CAD build for the part. Positions are in the model's coordinates, mm. Coordinates: 2 decimals unless noted, no trailing zeros. Loops run counter-clockwise (first coordinate to the right, second up) from the corner with the lowest first, then second, coordinate; pieces in that order, holes last. Notation, with made-up numbers: (66.25, -39) -> (114.25, -39) arc R28 cw to (114.25, -3) -> close; hole circle Ø2 at (50, 42.5). An arc over 180 degrees is marked (long way). Write each question's results on one line, items separated by ' | '.
from build123d import *

# Parameters (mm, degrees)
EXTRUDE_1_DEPTH          = 5
CUT_EXTRUDE_1_DEPTH      = 373.886350983
CUT_EXTRUDE_1_DEPTH_BACK = 373.886350983
CUT_EXTRUDE_2_REACH      = 374.886
SKETCH_4_W               = 120
SKETCH_4_H               = 360
FILLET_1_R               = 30


with BuildPart() as part:
    # 草图2 → 凸台-拉伸1 (new body)
    with BuildSketch(Plane(origin=(0, 0, 0), x_dir=(1, 0, 0), z_dir=(0, 1, 0))):
        Polygon((-197.790744863, 180), (-266.129914045, 63.779122951), (-81.97, -261.14), (81.97, -261.14), (266.129914045, 63.779122951), (197.790744863, 180), align=None)
    extrude(amount=EXTRUDE_1_DEPTH)

    # 草图3 → 切除-拉伸1 (cut, two sides: drawn at the far end of the back side and taken through both)
    with BuildSketch(Plane(origin=(0, 5, 0), x_dir=(1, 0, 0), z_dir=(0, 1, 0)).offset(-CUT_EXTRUDE_1_DEPTH_BACK)):
        Polygon((25, 95), (110, 180), (-110, 180), (-25, 95), align=None)
    extrude(amount=CUT_EXTRUDE_1_DEPTH + CUT_EXTRUDE_1_DEPTH_BACK, mode=Mode.SUBTRACT)

    # 草图4 → 切除-拉伸2 (cut, up to next)
    with BuildSketch(Plane(origin=(0, 5, 0), x_dir=(1, 0, 0), z_dir=(0, 1, 0)), mode=Mode.PRIVATE) as cut_extrude_2_sk1:
        with Locations((0, 65)):
            Rectangle(SKETCH_4_W, SKETCH_4_H)
    cut_extrude_2_tool1 = extrude(cut_extrude_2_sk1.sketch, amount=-CUT_EXTRUDE_2_REACH, mode=Mode.PRIVATE) & part.part
    add(cut_extrude_2_tool1.solids().sort_by_distance((0, 5, -65))[0], mode=Mode.SUBTRACT)

    # 圆角1
    fillet_1_edges = [part.edges().sort_by_distance(p)[0] for p in [
        (197.790744863, 2.5, -180),
        (266.129914045, 2.5, -63.779122951),
        (81.97, 2.5, 261.14),
        (-81.97, 2.5, 261.14),
        (-266.129914045, 2.5, -63.779122951),
        (-197.790744863, 2.5, -180),
    ]]
    fillet(fillet_1_edges, radius=FILLET_1_R)


solid = part.part
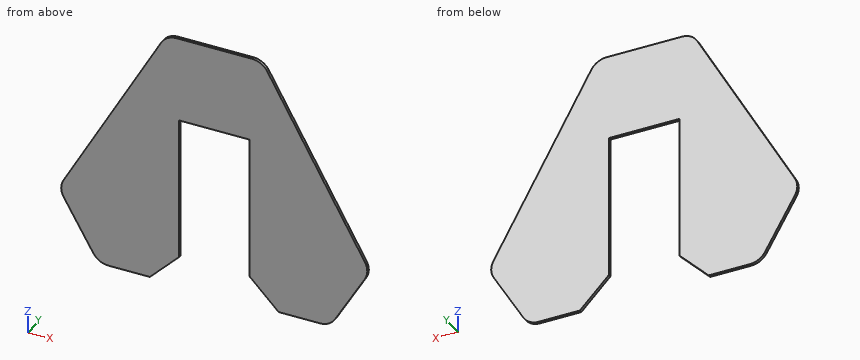
1) Slice it at D-D (z = -147). Write the cut outline in (x, y).
Outcome:
outline: (-217.2, 0) -> (-77, 0) -> (-77, 5) -> (-217.2, 5) -> close; (77, 0) -> (217.2, 0) -> (217.2, 5) -> (77, 5) -> close
2) Drill centre lines: L1, parallel to Z at x = -20, y = 3.45; L2, parallel to X at y = 3.3, z = -67; L3, parallel to X at y = 0.6, z = -149.5. Where is each one in solid material? Low to high. Write a range as from..to.
Outcome:
L1: z = 115..261.14 | L2: x = -261.29..-60, 60..261.29 | L3: x = -215.73..-79.5, 79.5..215.73
3) Slice it at A-A (z = 19.5). Write the cut outline in (x, y), then the cut area to 3 significant figures.
Outcome:
outline: (-218.93, 0) -> (-60, 0) -> (-60, 5) -> (-218.93, 5) -> close; (60, 0) -> (218.93, 0) -> (218.93, 5) -> (60, 5) -> close | area: 1,590 mm^2
4) Pin check, flat tips, straight feed: pin 1 (1 mm diameter, centred on y = 2, z = 113.5, fed in from -X); pin 2 (1.5 mm diameter, centred on x = 4.5, z = 208, fed in from -Y); pin 3 (1.5 mm diameter, centred on x = 28.5, y = 3.5, fed in from -Z). Stop position of each tip, or through.
Outcome:
pin 1: stops at x = -165.93 | pin 2: stops at y = 0 | pin 3: stops at z = 115
5) Slice it at C-C (x = -189). Write the cut outline in (y, z).
Outcome:
outline: (0, -178.81) -> (5, -178.81) -> (5, 72.3) -> (0, 72.3) -> close
6) Slice it at B-B (y = 2.7). Write the cut outline in (x, z).
Outcome:
outline: (-257.59, -48.71) arc R30 ccw to (-257.35, -78.71) -> (-206.49, -165.21) arc R30 ccw to (-180.63, -180) -> (-110, -180) -> (-60, -130) -> (-60, 115) -> (60, 115) -> (60, -130) -> (110, -180) -> (180.63, -180) arc R30 ccw to (206.49, -165.21) -> (257.35, -78.71) arc R30 ccw to (257.59, -48.71) -> (90.59, 245.93) arc R30 ccw to (64.49, 261.14) -> (-64.49, 261.14) arc R30 ccw to (-90.59, 245.93) -> close
